Print and shaded views of the part. All mm, measured from the part's lowest x, y and z. Round coordinates to 2 decimals unless told otherwise and drop trailing zeros. Write each loop counter-clockwise with the first axis right and the second up, starting at its lowest first coordinate (ties: lowest second). Pieces come first, ordered by that corner, then holes. Notation, with made-up numbers: (49, 5) - (78, 5) arc R29 cw to (78, 43) - close; hole circle Ø2 at (69.5, 42.5). An arc over 180 degrees is marked (long way). One line per item, written item: value.
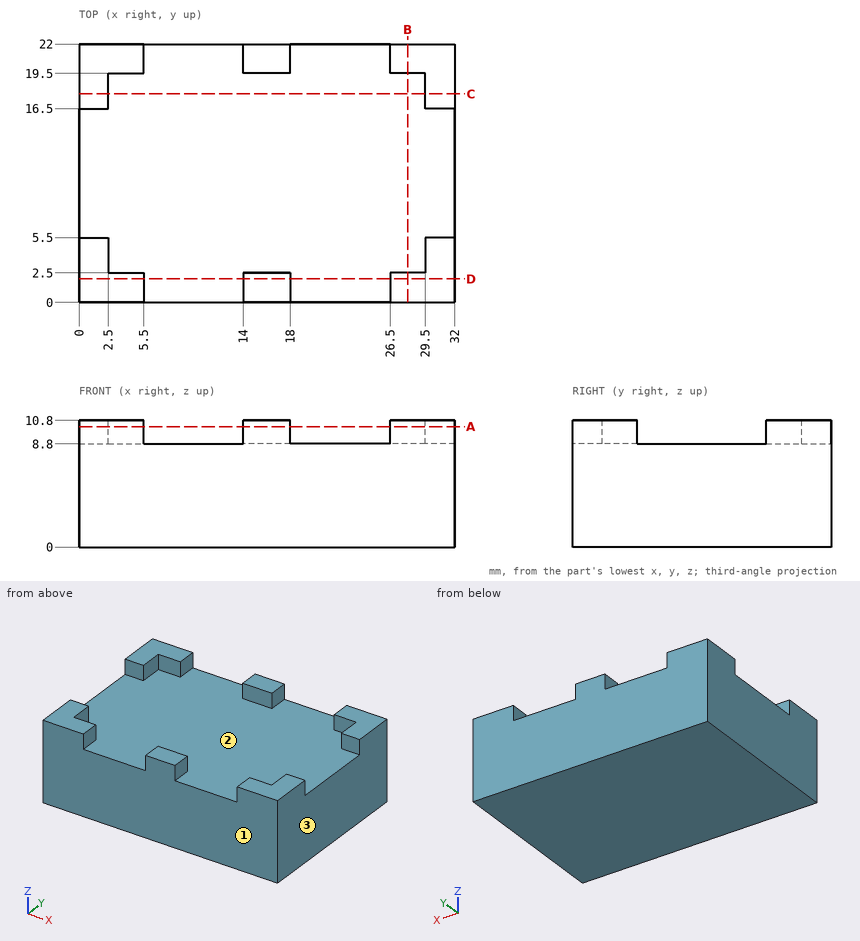
1. Band-saw the part on D-D on y = 2. Write the cut outline in (x, z).
Report:
outline: (0, 0) - (32, 0) - (32, 10.8) - (26.5, 10.8) - (26.5, 8.8) - (18, 8.8) - (18, 10.8) - (14, 10.8) - (14, 8.8) - (5.5, 8.8) - (5.5, 10.8) - (0, 10.8) - close
2. Band-saw the part on A-A on z = 10.25. State how many separate pieces and enclosed holes the cut face has, plus the area to 3 significant figures.
Report:
separate pieces: 6
enclosed holes: 0
area: 105 mm²
3. Mould opens along X. For the marked faces 1, 2 and 3 say: released by +X, released by -X, zero draft, split by the parting line, or undercut.
Report:
face 1: zero draft
face 2: undercut
face 3: released by +X
4. Wall check: probe 1 along X at (y, z) = (1.75, 10.25); probe 2 along Z at (x, y) = (28.5, 12.5). Give the ranges that are in metal, low to high. Write a range as [from, to].
Report:
probe 1: [0, 5.5], [14, 18], [26.5, 32]
probe 2: [0, 8.8]
5. Band-saw the part on C-C on y = 17.75. Write the cut outline in (x, z).
Report:
outline: (0, 0) - (32, 0) - (32, 10.8) - (29.5, 10.8) - (29.5, 8.8) - (2.5, 8.8) - (2.5, 10.8) - (0, 10.8) - close
6. Drop a flat-ended pin along its axis: pin 1 (6 mm diameter, centred on x = 9.5, y = 13.5, fed in from +Z). Give the stop position or say it passes through.
Report:
pin 1: z = 8.8
7. Band-saw the part on B-B on x = 28. Write the cut outline in (y, z).
Report:
outline: (0, 0) - (22, 0) - (22, 10.8) - (19.5, 10.8) - (19.5, 8.8) - (2.5, 8.8) - (2.5, 10.8) - (0, 10.8) - close
